Work out the finished part from the listing and answer in its coordinate system (mm). A direction names the side the tool comes from. Give positions to 0.01 mm unless a question says otherwise; leave off trailing zeros. Loops run counter-clockwise (first coordinate to the right, second up) from the corner with the lowest first, then second, coordinate; pieces in that order, holes last. Notation, with made-up numbers: (58, 13.25) - (101, 13.25) arc R14 ccw to (101, 20.25) - close; hole circle Ø6 at (82.25, 3.5). An arc over 180 degrees is marked (long way). One line per question, with ' | ' between items. Start each with the question number.
1. Which of the six approach directions +Z, -Z, +X, -X, +Y, -Y give full straight-line access (tool end or side, diameter ignored) to faces 1 (the face through (35, 0, -22)), 2 (the face through (38, -15.875, -11)), 3 (the face through (35, 0, 22)), 4 (the face through (34.273, 7.76, -0.692))?
2. Section C-C (y = -25.5) is taken. Determine the outline of the cut face in (x, z), plus the area to 3 significant figures.
3. For a pull along Z with two mould halves and no side action, classify faces 5 (the face through (50, 20.638, 0)), 6 (the face through (-47.613, -10.397, -1.047)), 7 (the face through (-29.133, -2.348, -37.28)) as released by +Z, released by -Z, zero draft, split by the parting line, or undercut.
4. Find the intervals of material crossed by line 1 (Y direction, x = 35.5, z = 18.5) (3 decimals); line 2 (Y direction, x = -24, z = 14.5); line 3 (X direction, y = 1.5, z = -9), in increasing order.
5. Each of these flat-tipped pins is pushed along its axis until it touches: pin 1 (10 mm diameter, centred on x = 42.5, y = -1.5, fed in from -Z); pin 2 (6 mm diameter, centred on y = 7, z = -13.5, fed in from -X); pin 3 (12 mm diameter, centred on x = 46, z = -18.5, fed in from -Y) (3 decimals). Where does it stop, or does it pass through?
6. Section D-D (z = 36) is taken. Determine the outline of the cut face in (x, y) (1 decimal), plus the area to 3 significant figures.
from build123d import *

# Parameters (mm, degrees)
BOSS_EXTRUDE1_START = -15.875
SKETCH1_R           = 38.89375
BOSS_EXTRUDE1_DEPTH = 17.4625
BOSS_EXTRUDE2_START = 15.875
BOSS_EXTRUDE2_DEPTH = 11.1125
BOSS_EXTRUDE3_REACH = 89.863
SKETCH3_R           = 4.5
SKETCH4_R           = 15.748
BOSS_EXTRUDE4_DEPTH = 25.4


with BuildPart() as part:
    # Sketch1 → Boss-Extrude1 (new body)
    with BuildSketch(Plane(origin=(0, 0, 0), x_dir=(1, 0, 0), z_dir=(0, 1, 0)).offset(BOSS_EXTRUDE1_START)):
        Circle(SKETCH1_R)
    extrude(amount=-BOSS_EXTRUDE1_DEPTH)

    # Sketch2 → Boss-Extrude2 (add)
    with BuildSketch(Plane(origin=(0, 0, 0), x_dir=(-1, 0, 0), z_dir=(0, -1, 0)).offset(BOSS_EXTRUDE2_START)):
        with BuildLine():
            Line((-58.018619526, 13.704654669), (0, 47.625))
            ThreePointArc((0, 47.625), (47.625, 0), (0, -47.625))
            Line((0, -47.625), (-58.018619526, -13.704654669))
            ThreePointArc((-58.018619526, -13.704654669), (-65.88125, 0), (-58.018619526, 13.704654669))
        make_face()
    extrude(amount=-BOSS_EXTRUDE2_DEPTH)

    # Sketch3 → Boss-Extrude3 (add, up to next)
    with BuildSketch(Plane(origin=(0, 0, 0), x_dir=(-1, 0, 0), z_dir=(0, -1, 0)), mode=Mode.PRIVATE) as boss_extrude3_sk1:
        with Locations(Location((-35.208032093, 21.828125, 0), (0, 0, 120.312514276))):
            Circle(SKETCH3_R)
    boss_extrude3_tool1 = extrude(boss_extrude3_sk1.sketch, amount=BOSS_EXTRUDE3_REACH, mode=Mode.PRIVATE) - part.part
    # Sketch3 → Boss-Extrude3 (add, up to next)
    with BuildSketch(Plane(origin=(0, 0, 0), x_dir=(-1, 0, 0), z_dir=(0, -1, 0)), mode=Mode.PRIVATE) as boss_extrude3_sk2:
        with Locations(Location((-35.208032093, -21.828125, 0), (0, 0, 239.687485724))):
            Circle(SKETCH3_R)
    boss_extrude3_tool2 = extrude(boss_extrude3_sk2.sketch, amount=BOSS_EXTRUDE3_REACH, mode=Mode.PRIVATE) - part.part
    # Sketch3 → Boss-Extrude3 (add, up to next)
    with BuildSketch(Plane(origin=(0, 0, 0), x_dir=(-1, 0, 0), z_dir=(0, -1, 0)), mode=Mode.PRIVATE) as boss_extrude3_sk3:
        with Locations(Location((25.298418923, -34.925, 0), (0, 0, 305.918677721))):
            Circle(SKETCH3_R)
    boss_extrude3_tool3 = extrude(boss_extrude3_sk3.sketch, amount=BOSS_EXTRUDE3_REACH, mode=Mode.PRIVATE) - part.part
    # Sketch3 → Boss-Extrude3 (add, up to next)
    with BuildSketch(Plane(origin=(0, 0, 0), x_dir=(-1, 0, 0), z_dir=(0, -1, 0)), mode=Mode.PRIVATE) as boss_extrude3_sk4:
        with Locations(Location((25.298418923, 34.925, 0), (0, 0, 54.082225764))):
            Circle(SKETCH3_R)
    boss_extrude3_tool4 = extrude(boss_extrude3_sk4.sketch, amount=BOSS_EXTRUDE3_REACH, mode=Mode.PRIVATE) - part.part
    add(boss_extrude3_tool1.solids().sort_by_distance((35.208032, 0, -21.828125))[0])
    add(boss_extrude3_tool2.solids().sort_by_distance((35.208032, 0, 21.828125))[0])
    add(boss_extrude3_tool3.solids().sort_by_distance((-25.298419, 0, 34.925))[0])
    add(boss_extrude3_tool4.solids().sort_by_distance((-25.298419, 0, -34.925))[0])

    # Sketch4 → Boss-Extrude4 (add)
    with BuildSketch(Plane(origin=(0, -4.7625, 0), x_dir=(1, 0, 0), z_dir=(0, 1, 0))):
        with Locations((50.00625, 0)):
            Circle(SKETCH4_R)
    extrude(amount=BOSS_EXTRUDE4_DEPTH)


solid = part.part
Conclusion:
1) face 1: -Z, +X, -X, +Y | face 2: -Y | face 3: +Z, +X, -X, +Y | face 4: +Y
2) outline: circle Ø77.79 at (0, 0) | area: 4,750 mm²
3) face 5: zero draft | face 6: split by the parting line | face 7: undercut
4) line 1: -15.875 to 0 | line 2: -33.34 to -4.76 | line 3: 37.08 to 62.93
5) pin 1: z = -25.7 | pin 2: x = 38.27 | pin 3: y = -15.875
6) outline: (-31.2, -15.9) - (-14.7, -15.9) - (-14.7, -33.3) - (14.7, -33.3) - (14.7, -15.9) - (19.9, -15.9) - (19.9, -4.8) - (-20.9, -4.8) - (-20.9, 0) - (-29.7, 0) - (-29.7, -4.8) - (-31.2, -4.8) - close | area: 1,120 mm²
